Input: dimensioned drawing with shaded views. Units: mm. Origin: part minimum x, y, z. A direction names the side the tool comes from. Coordinates: 2 decimals unless noted, no trailing zeros. Loops run counter-clockwise (first coordinate to the right, second up) from the corner with the lowest first, then second, coordinate; pieces in that order, holes last. Notation, with made-up numbers: M 3,32 L 30,32 A25 ccw 30,50 Z; hole C -5.75,-12.75 d8. An arc over 180 degrees is marked long. Write item = value, one per line. Start each with the question number.
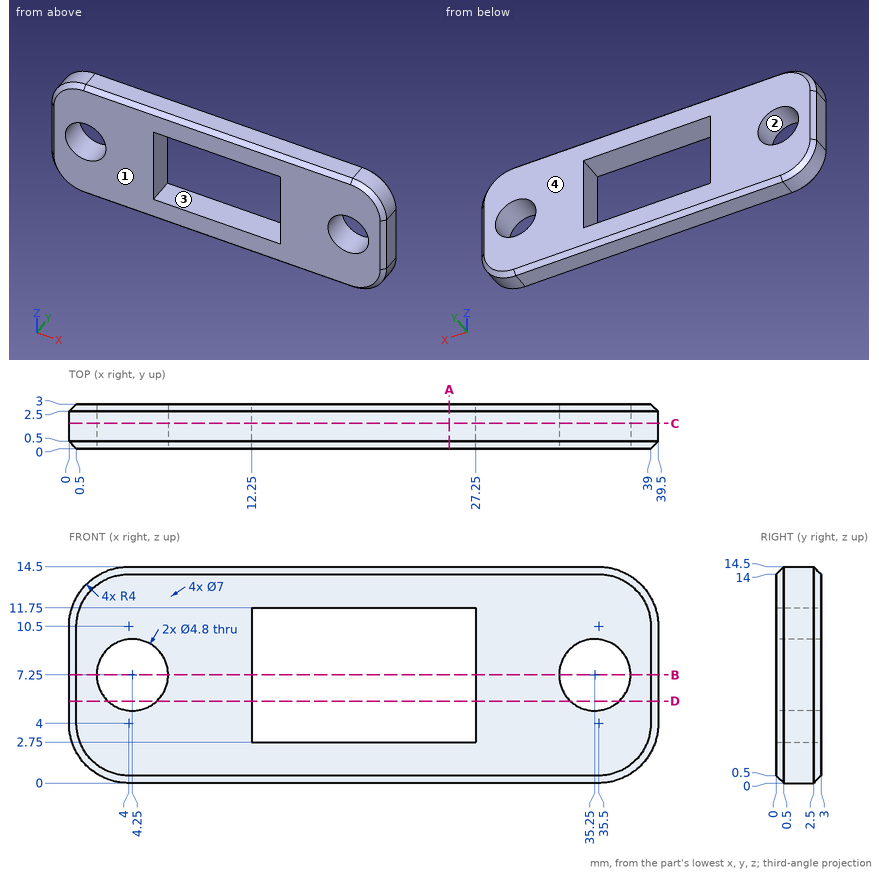
Item 1: Section query B-B (z = 7.25). Return the cut outline in (x, y), plus the area to 3 significant figures.
Item 2: Pull-direction query (Z, two-part tool) for the marked faces 1 and 2; classes: released by +Z, released by -Z, zero draft, split by the parting line, or undercut.
Item 3: Section query A-A (x = 25.5). Return the cut outline in (y, z), plus the area to 3 significant figures.
Item 4: Section query D-D (z = 5.5). Return the cut outline in (x, y), plus the area to 3 significant figures.
Item 5: Reachability of the marked faces 3 and 4 from +Z, -Z, +X, -X, +Y, -Y: full face, straight path, thin tool, end or side. Return the list, or none.
Item 6: Section query C-C (y = 1.7). Return the cut outline in (x, z), plus the area to 3 significant figures.
Item 7: Line query: line 1 (Z direction, x = 20.5, y = 0.5); line 2 (X direction, y = 0.8, z = 4.5); line 3 (Z direction, x = 4.25, y = 1.3). Output: solid intervals per line, ascending. Write a range as from..to.
Item 8: First-contact query: pin 1 (1.5 mm diameter, centred on y = 0.5, z = 3, fed in from +X); pin 2 (3 mm diameter, centred on x = 4.25, z = 7.25, fed in from -Y). Flat tips, straight axial feed; report the tip coordinate or a pass-through.
Verdict:
q1.outline = M 0,0.5 L 0.5,0 L 1.85,0 L 1.85,3 L 0.5,3 L 0,2.5 Z; M 6.65,0 L 12.25,0 L 12.25,3 L 6.65,3 Z; M 27.25,0 L 32.85,0 L 32.85,3 L 27.25,3 Z; M 37.65,0 L 39,0 L 39.5,0.5 L 39.5,2.5 L 39,3 L 37.65,3 Z
q1.area = 44.2 mm2
q2.face_1 = zero draft
q2.face_2 = undercut
q3.outline = M 0,0.5 L 0.5,0 L 2.5,0 L 3,0.5 L 3,2.75 L 0,2.75 Z; M 0,11.75 L 3,11.75 L 3,14 L 2.5,14.5 L 0.5,14.5 L 0,14 Z
q3.area = 16.0 mm2
q4.outline = M 0,0.5 L 0.5,0 L 2.61,0 L 2.61,3 L 0.5,3 L 0,2.5 Z; M 5.89,0 L 12.25,0 L 12.25,3 L 5.89,3 Z; M 27.25,0 L 33.61,0 L 33.61,3 L 27.25,3 Z; M 36.89,0 L 39,0 L 39.5,0.5 L 39.5,2.5 L 39,3 L 36.89,3 Z
q4.area = 53.3 mm2
q5.face_3 = +Y, -Y
q5.face_4 = +Z, -Z, +X, -X, +Y
q6.outline = M 0,4 A4 ccw 4,0 L 35.5,0 A4 ccw 39.5,4 L 39.5,10.5 A4 ccw 35.5,14.5 L 4,14.5 A4 ccw 0,10.5 Z; hole C 4.25,7.25 d4.8; hole M 12.25,2.75 L 27.25,2.75 L 27.25,11.75 L 12.25,11.75 Z; hole C 35.25,7.25 d4.8
q6.area = 388 mm2
q7.line_1 = 0..2.75, 11.75..14.5
q7.line_2 = 0..12.25, 27.25..39.5
q7.line_3 = 0..4.85, 9.65..14.5
q8.pin_1 = 39.49
q8.pin_2 = through
